Read the model definition and answer for the solid it produces. Units are mm, in the model's axes. Face numbers are marked on the shaded views. Round coordinates to 2 decimals unless told otherwise and drop trailing zeros. Order: outer loops, then holes, each group sorted by start corner. A loop starts at its lowest first (then second) coordinate and runs counter-clockwise, first axis right, second up.
from build123d import *

# Parameters (mm, degrees)
F0_R     = 17.65
F0_R_2   = 16.65
F1_DEPTH = 15.5
F2_DEPTH = 101
F2_TAPER = 3
F3_R     = 2
F4_D     = 8
F4_DEPTH = 90
F4_TIP   = 2.4034424761


with BuildPart() as f1:
    # F0 (on Top) → F1 (new body)
    with BuildSketch(Plane.XY):
        Circle(F0_R)
        Circle(F0_R_2, mode=Mode.SUBTRACT)
    extrude(amount=F1_DEPTH)

    # F0 (on Top) → F2 (join)
    with BuildSketch(Plane.XY):
        Circle(F0_R)
        Circle(F0_R_2, mode=Mode.SUBTRACT)
        Circle(F0_R_2)
    extrude(amount=-F2_DEPTH, taper=F2_TAPER)

    # F3
    f3_edges = [f1.edges().sort_by_distance(p)[0] for p in [
        (-12.356814, 0, -101),
    ]]
    fillet(f3_edges, radius=F3_R)

    # F4
    with Locations(Plane.XY):
        with Locations((0, 0)):
            Hole(F4_D / 2, depth=F4_DEPTH)
            with Locations((0, 0, -(F4_DEPTH + F4_TIP / 2))):  # 118° drill point
                Cone(0, F4_D / 2, F4_TIP, mode=Mode.SUBTRACT)


solid = f1.part
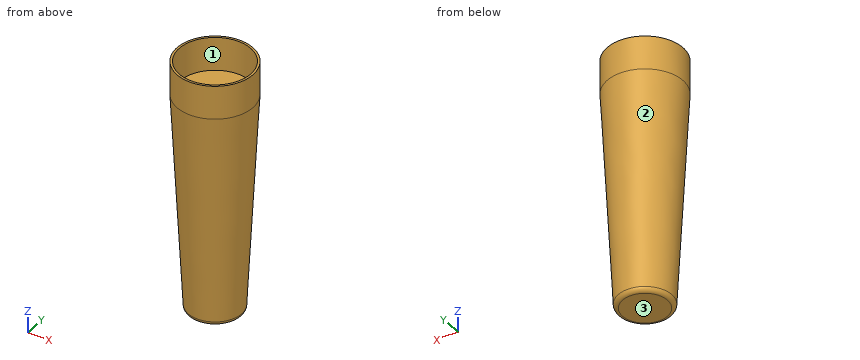
Q1. A cutting plane is placed at A-A, the plane z = -2.5. Give the vertices of the cut face in (x, y), plus the area to 3 significant figures.
Outcome:
outline: circle Ø35.04 at (0, 0); hole circle Ø8 at (0, 0)
area: 914 mm2
Q2. Straight lines are drawn through the part: probe 1 along Y at (x, z) = (0, 10); probe 2 along Z at (x, y) = (6.5, -1); probe 3 along X at (y, z) = (0, -50). For each, find the intervals that lie inside material, in ascending order.
Outcome:
probe 1: y = -17.65 to -16.65, 16.65 to 17.65
probe 2: z = -101 to 0
probe 3: x = -15.03 to -4, 4 to 15.03
Q3. Flat-ended cylindrical pins translate along their axes: pin 1 (4 mm diameter, centred on x = -2, z = -34, fed in from -Y); pin 2 (3 mm diameter, centred on x = 9, z = -82, fed in from +Y); pin 3 (1 mm diameter, centred on x = -10.5, z = -5, fed in from +Y). Find the tip coordinate at first contact, or state that the pin passes through.
Outcome:
pin 1: stops at y = -15.93
pin 2: stops at y = 11.05
pin 3: stops at y = 14.23
Q4. A cutting plane is placed at C-C, the plane z = -36. Give the vertices of the cut face in (x, y), plus the area to 3 significant figures.
Outcome:
outline: circle Ø31.53 at (0, 0); hole circle Ø8 at (0, 0)
area: 730 mm2
Q5. For a pull along Y with two mould halves and no side action, classify the marked faces 1, 2 and 3 as released by +Y, released by -Y, zero draft, split by the parting line, or undercut.
Outcome:
face 1: undercut
face 2: split by the parting line
face 3: zero draft
Q6. A cutting plane is placed at B-B, the plane z = -93.5. Give the vertices of the cut face in (x, y), plus the area to 3 significant figures.
Outcome:
outline: circle Ø25.5 at (0, 0)
area: 511 mm2
